```python
from build123d import *

# Parameters (mm, degrees)
SKETCH_1_W      = 42
SKETCH_1_H      = 3
SKETCH_1_H_2    = 42
SKETCH_1_R      = 1.6
SKETCH_1_R_2    = 4.5
SKETCH_1_H_3    = 10
EXTRUDE_1_DEPTH = 6


with BuildPart() as part:
    # 草图1 → 凸台-拉伸1 (new body)
    # profile 1 of 18: a face of its own
    with BuildSketch(Plane.XY):
        with Locations((0, 43.5)):
            Rectangle(SKETCH_1_W, SKETCH_1_H)
    # profile 2 of 18: a face of its own
    with BuildSketch(Plane.XY):
        with BuildLine():
            Line((21, 92), (-21, 92))
            Line((-21, 92), (-16.63137085, 87.63137085))
            ThreePointArc((-16.63137085, 87.63137085), (-15.129338595, 88.056473618), (-13.980131585, 87))
            Line((-13.980131585, 87), (13.980131585, 87))
            ThreePointArc((13.980131585, 87), (15.5, 88.1), (17.019868415, 87))
            Line((17.019868415, 87), (21, 87))
            Line((21, 87), (21, 92))
        make_face()
    # profile 3 of 18: a face of its own
    with BuildSketch(Plane.XY):
        with BuildLine():
            Line((-21, 92), (-21, 87))
            Line((-21, 87), (-17.019868415, 87))
            ThreePointArc((-17.019868415, 87), (-16.862690243, 87.338495857), (-16.63137085, 87.63137085))
            Line((-16.63137085, 87.63137085), (-21, 92))
        make_face()
    # profile 4 of 18: a face of its own
    with BuildSketch(Plane.XY):
        with BuildLine():
            Line((-17.019868415, 87), (-21, 87))
            Line((-21, 87), (-17.1, 83.1))
            Line((-17.1, 83.1), (-17.1, 86.5))
            ThreePointArc((-17.1, 86.5), (-17.079840097, 86.753190181), (-17.019868415, 87))
        make_face()
    # profile 5 of 18: a face of its own
    with BuildSketch(Plane.XY):
        with BuildLine():
            Line((13.980131585, 87), (-13.980131585, 87))
            ThreePointArc((-13.980131585, 87), (-13.920159903, 86.753190181), (-13.9, 86.5))
            Line((-13.9, 86.5), (-13.9, 84.9))
            Line((-13.9, 84.9), (-1.767766953, 72.767766953))
            ThreePointArc((-1.767766953, 72.767766953), (0.956708581, 73.309698831), (2.5, 71))
            Line((2.5, 71), (2.5, 68.5))
            Line((2.5, 68.5), (14.36862915, 56.63137085))
            ThreePointArc((14.36862915, 56.63137085), (16.112293492, 56.978207252), (17.1, 55.5))
            Line((17.1, 55.5), (17.1, 53.9))
            Line((17.1, 53.9), (21, 50))
            Line((21, 50), (21, 87))
            Line((21, 87), (17.019868415, 87))
            ThreePointArc((17.019868415, 87), (17.079840097, 86.753190181), (17.1, 86.5))
            Line((17.1, 86.5), (17.1, 81.5))
            ThreePointArc((17.1, 81.5), (15.5, 79.9), (13.9, 81.5))
            Line((13.9, 81.5), (13.9, 86.5))
            ThreePointArc((13.9, 86.5), (13.920159903, 86.753190181), (13.980131585, 87))
        make_face()
    # profile 6 of 18: a face of its own
    with BuildSketch(Plane.XY):
        with BuildLine():
            ThreePointArc((-13.9, 81.5), (-14.021792748, 80.887706508), (-14.36862915, 80.36862915))
            Line((-14.36862915, 80.36862915), (-2.5, 68.5))
            Line((-2.5, 68.5), (-2.5, 71))
            ThreePointArc((-2.5, 71), (-2.309698831, 71.956708581), (-1.767766953, 72.767766953))
            Line((-1.767766953, 72.767766953), (-13.9, 84.9))
            Line((-13.9, 84.9), (-13.9, 81.5))
        make_face()
    # profile 7 of 18: a face of its own
    with BuildSketch(Plane.XY):
        with BuildLine():
            Line((-17.1, 83.1), (-21, 87))
            Line((-21, 87), (-21, 50))
            Line((-21, 50), (-17.019868415, 50))
            ThreePointArc((-17.019868415, 50), (-17.079840097, 50.246809819), (-17.1, 50.5))
            Line((-17.1, 50.5), (-17.1, 55.5))
            ThreePointArc((-17.1, 55.5), (-15.5, 57.1), (-13.9, 55.5))
            Line((-13.9, 55.5), (-13.9, 50.5))
            ThreePointArc((-13.9, 50.5), (-13.920159903, 50.246809819), (-13.980131585, 50))
            Line((-13.980131585, 50), (13.980131585, 50))
            ThreePointArc((13.980131585, 50), (13.920159903, 50.246809819), (13.9, 50.5))
            Line((13.9, 50.5), (13.9, 52.1))
            Line((13.9, 52.1), (1.767766953, 64.232233047))
            ThreePointArc((1.767766953, 64.232233047), (-0.956708581, 63.690301169), (-2.5, 66))
            Line((-2.5, 66), (-2.5, 68.5))
            Line((-2.5, 68.5), (-14.36862915, 80.36862915))
            ThreePointArc((-14.36862915, 80.36862915), (-16.112293492, 80.021792748), (-17.1, 81.5))
            Line((-17.1, 81.5), (-17.1, 83.1))
        make_face()
    # profile 8 of 18: a face of its own
    with BuildSketch(Plane.XY):
        with BuildLine():
            ThreePointArc((2.5, 66), (2.309698831, 65.043291419), (1.767766953, 64.232233047))
            Line((1.767766953, 64.232233047), (13.9, 52.1))
            Line((13.9, 52.1), (13.9, 55.5))
            ThreePointArc((13.9, 55.5), (14.021792748, 56.112293492), (14.36862915, 56.63137085))
            Line((14.36862915, 56.63137085), (2.5, 68.5))
            Line((2.5, 68.5), (2.5, 66))
        make_face()
    # profile 9 of 18: a face of its own
    with BuildSketch(Plane.XY):
        with BuildLine():
            Line((17.019868415, 50), (21, 50))
            Line((21, 50), (17.1, 53.9))
            Line((17.1, 53.9), (17.1, 50.5))
            ThreePointArc((17.1, 50.5), (17.079840097, 50.246809819), (17.019868415, 50))
        make_face()
    # profile 10 of 18: a face of its own
    with BuildSketch(Plane.XY):
        with BuildLine():
            Line((16.63137085, 49.36862915), (21, 45))
            Line((21, 45), (21, 50))
            Line((21, 50), (17.019868415, 50))
            ThreePointArc((17.019868415, 50), (16.862690243, 49.661504143), (16.63137085, 49.36862915))
        make_face()
    # profile 11 of 18: a face of its own
    with BuildSketch(Plane.XY):
        with BuildLine():
            Line((-17.019868415, 50), (-21, 50))
            Line((-21, 50), (-21, 45))
            Line((-21, 45), (21, 45))
            Line((21, 45), (16.63137085, 49.36862915))
            ThreePointArc((16.63137085, 49.36862915), (15.129338595, 48.943526382), (13.980131585, 50))
            Line((13.980131585, 50), (-13.980131585, 50))
            ThreePointArc((-13.980131585, 50), (-15.5, 48.9), (-17.019868415, 50))
        make_face()
    # profile 12 of 18: a face of its own
    with BuildSketch(Plane.XY):
        with Locations((0, 43.5)):
            Rectangle(SKETCH_1_W, SKETCH_1_H)
    # profile 13 of 18: a face of its own
    with BuildSketch(Plane.XY):
        with Locations((0, 21)):
            Rectangle(SKETCH_1_W, SKETCH_1_H_2)
        with Locations((-15.5, 5.5)):
            Circle(SKETCH_1_R, mode=Mode.SUBTRACT)
        with Locations((15.5, 5.5)):
            Circle(SKETCH_1_R, mode=Mode.SUBTRACT)
        with Locations((-15.5, 36.5)):
            Circle(SKETCH_1_R, mode=Mode.SUBTRACT)
        with Locations((0, 21)):
            Circle(SKETCH_1_R_2, mode=Mode.SUBTRACT)
        with Locations((15.5, 36.5)):
            Circle(SKETCH_1_R, mode=Mode.SUBTRACT)
    # profile 14 of 18: a face of its own
    with BuildSketch(Plane.XY):
        with Locations((0, -5)):
            Rectangle(SKETCH_1_W, SKETCH_1_H_3)
    # profile 15 of 18: a face of its own
    with BuildSketch(Plane.XY):
        with BuildLine():
            Line((21, -10), (-21, -10))
            Line((-21, -10), (-16.63137085, -14.36862915))
            ThreePointArc((-16.63137085, -14.36862915), (-14.887706508, -14.021792748), (-13.9, -15.5))
            ThreePointArc((-13.9, -15.5), (-14.021792748, -16.112293492), (-14.36862915, -16.63137085))
            Line((-14.36862915, -16.63137085), (-1.060660172, -29.939339828))
            ThreePointArc((-1.060660172, -29.939339828), (0, -29.5), (1.060660172, -29.939339828))
            Line((1.060660172, -29.939339828), (14.36862915, -16.63137085))
            ThreePointArc((14.36862915, -16.63137085), (14.36862915, -14.36862915), (16.63137085, -14.36862915))
            Line((16.63137085, -14.36862915), (21, -10))
        make_face()
    # profile 16 of 18: a face of its own
    with BuildSketch(Plane.XY):
        with BuildLine():
            Line((-16.63137085, -14.36862915), (-21, -10))
            Line((-21, -10), (-21, -52))
            Line((-21, -52), (-16.63137085, -47.63137085))
            ThreePointArc((-16.63137085, -47.63137085), (-16.63137085, -45.36862915), (-14.36862915, -45.36862915))
            Line((-14.36862915, -45.36862915), (-1.060660172, -32.060660172))
            ThreePointArc((-1.060660172, -32.060660172), (-1.5, -31), (-1.060660172, -29.939339828))
            Line((-1.060660172, -29.939339828), (-14.36862915, -16.63137085))
            ThreePointArc((-14.36862915, -16.63137085), (-16.63137085, -16.63137085), (-16.63137085, -14.36862915))
        make_face()
    # profile 17 of 18: a face of its own
    with BuildSketch(Plane.XY):
        with BuildLine():
            Line((-16.63137085, -47.63137085), (-21, -52))
            Line((-21, -52), (21, -52))
            Line((21, -52), (16.63137085, -47.63137085))
            ThreePointArc((16.63137085, -47.63137085), (14.36862915, -47.63137085), (14.36862915, -45.36862915))
            Line((14.36862915, -45.36862915), (1.060660172, -32.060660172))
            ThreePointArc((1.060660172, -32.060660172), (0, -32.5), (-1.060660172, -32.060660172))
            Line((-1.060660172, -32.060660172), (-14.36862915, -45.36862915))
            ThreePointArc((-14.36862915, -45.36862915), (-14.021792748, -45.887706508), (-13.9, -46.5))
            ThreePointArc((-13.9, -46.5), (-14.887706508, -47.978207252), (-16.63137085, -47.63137085))
        make_face()
    # profile 18 of 18: a face of its own
    with BuildSketch(Plane.XY):
        with BuildLine():
            Line((21, -52), (21, -10))
            Line((21, -10), (16.63137085, -14.36862915))
            ThreePointArc((16.63137085, -14.36862915), (16.978207252, -14.887706508), (17.1, -15.5))
            ThreePointArc((17.1, -15.5), (16.112293492, -16.978207252), (14.36862915, -16.63137085))
            Line((14.36862915, -16.63137085), (1.060660172, -29.939339828))
            ThreePointArc((1.060660172, -29.939339828), (1.385819299, -30.425974851), (1.5, -31))
            ThreePointArc((1.5, -31), (1.385819299, -31.574025149), (1.060660172, -32.060660172))
            Line((1.060660172, -32.060660172), (14.36862915, -45.36862915))
            ThreePointArc((14.36862915, -45.36862915), (16.112293492, -45.021792748), (17.1, -46.5))
            ThreePointArc((17.1, -46.5), (16.978207252, -47.112293492), (16.63137085, -47.63137085))
            Line((16.63137085, -47.63137085), (21, -52))
        make_face()
    extrude(amount=EXTRUDE_1_DEPTH)


solid = part.part
```
The listing builds one solid part. Answer for the finished solid, in the listing's coordinates (mm). A direction names the side the tool comes from. Round coordinates to 2 decimals unless told otherwise and drop trailing zeros. Loops run counter-clockwise (first coordinate to the right, second up) from the corner with the lowest first, then second, coordinate; pieces in that order, holes last. Notation, with made-up numbers: (47.25, 33.25) - (94.25, 33.25) arc R25 ccw to (94.25, 62.25) - close; hole circle Ø2 at (-22, -29). An arc over 180 degrees is marked (long way). Return JSON: item names as keys, results as strings. Group by question number.
1. This flat-tipped pin is pushed along its axis until it touches: P1, Ø10, axis at x = 14, y = 55.5, coming from the -Z side. Where does it stop, or does it pass through?
2. Consider probe 1 along Y at (x, z) = (0, 3.75); probe 2 along X at (y, z) = (37.5, 5.6); probe 3 along Y at (x, z) = (1, 2.75). Determine where each line is inside the solid, lowest interval first.
3. Which of the six approach directions +Z, -Z, +X, -X, +Y, -Y give full straight-line access (tool end or side, diameter ignored) to faces 4 (the cylindrical face through (-15.5, 57.1, 3)), 5 (the flat face through (-5, 21, 0))?
4. The part is cut by section B-B on y = 36.5. Determine the outline of the cut face in (x, z), then the cut area to 3 significant figures.
5. The part is cut by section C-C on z = 4. State how many separate pieces and enclosed holes the cut face has, then the cut area to 3 significant figures.
6. The part is cut by section D-D on y = 21. Determine the outline of the cut face in (x, z), then the cut area to 3 significant figures.
7. The part is cut by section A-A on y = 69. Determine the outline of the cut face in (x, z), then the cut area to 3 significant figures.
8. The mould has two halves that part along Y. Classify faces 1 (the flat face through (0, 92, 3)), 2 (the cylindrical face through (15.5, 79.9, 3)), 3 (the flat face through (0, -52, 3)): pulls with the +Y half, pulls with the -Y half, needs draft (parallel to the pull), parting line crosses it, or undercut.
Resolved:
{
 "1": {"P1": "stops at z = 0"},
 "2": {"probe 1": "y = -52 to -32.5, -29.5 to 16.5, 25.5 to 63.5, 73.5 to 92", "probe 2": "x = -21 to -16.75, -14.25 to 14.25, 16.75 to 21", "probe 3": "y = -52 to -32.12, -29.88 to 16.61, 25.39 to 63.71, 73.29 to 92"},
 "3": {"face 4": "+Z, -Z", "face 5": "-Z, +X, -X, +Y, -Y"},
 "4": {"outline": "(-21, 0) - (-17.1, 0) - (-17.1, 6) - (-21, 6) - close; (-13.9, 0) - (13.9, 0) - (13.9, 6) - (-13.9, 6) - close; (17.1, 0) - (21, 0) - (21, 6) - (17.1, 6) - close", "area": "214 mm²"},
 "5": {"separate pieces": "1", "enclosed holes": "15", "area": "5,770 mm²"},
 "6": {"outline": "(-21, 0) - (-4.5, 0) - (-4.5, 6) - (-21, 6) - close; (4.5, 0) - (21, 0) - (21, 6) - (4.5, 6) - close", "area": "198 mm²"},
 "7": {"outline": "(-21, 0) - (-2.5, 0) - (-2.5, 6) - (-21, 6) - close; (2.5, 0) - (21, 0) - (21, 6) - (2.5, 6) - close", "area": "222 mm²"},
 "8": {"face 1": "pulls with the +Y half", "face 2": "undercut", "face 3": "pulls with the -Y half"}
}
